```python
from build123d import *

# Parameters (mm, degrees)
SKETCH1_W           = 97.3
SKETCH1_H           = 47
BOSS_EXTRUDE1_DEPTH = 1.6
SKETCH2_W           = 12.310757006
SKETCH2_H           = 2.521357674
SKETCH2_W_2         = 11.997879532
BOSS_EXTRUDE2_DEPTH = 20
SKETCH3_R           = 1.016
SKETCH3_R_2         = 1.316
CUT_EXTRUDE3_DEPTH  = 2.6


with BuildPart() as part:
    # Sketch1 → Boss-Extrude1 (new body)
    with BuildSketch(Plane(origin=(0, 0, 0), x_dir=(1, 0, 0), z_dir=(0, 1, 0))):
        with Locations((48.65, -23.5)):
            Rectangle(SKETCH1_W, SKETCH1_H)
    extrude(amount=BOSS_EXTRUDE1_DEPTH)

    # Sketch2 → Boss-Extrude2 (add)
    with BuildSketch(Plane(origin=(0, 1.6, 0), x_dir=(1, 0, 0), z_dir=(0, 1, 0))):
        with Locations((17.456098962, -45.739321163)):
            Rectangle(SKETCH2_W, SKETCH2_H)
        with Locations((66.019073535, -45.739321163)):
            Rectangle(SKETCH2_W_2, SKETCH2_H)
    extrude(amount=BOSS_EXTRUDE2_DEPTH)

    # Sketch3 → Cut-Extrude3 (cut, through all)
    with BuildSketch(Plane(origin=(0, 1.6, 0), x_dir=(1, 0, 0), z_dir=(0, 1, 0))):
        with Locations((3.16, -3.81)):
            Circle(SKETCH3_R)
        with Locations((93.617, -3.81)):
            Circle(SKETCH3_R)
        with Locations((93.744, -43.916)):
            Circle(SKETCH3_R_2)
        with Locations((3.16, -43.916)):
            Circle(SKETCH3_R)
    extrude(amount=-CUT_EXTRUDE3_DEPTH, mode=Mode.SUBTRACT)


solid = part.part
```
Check sheet for the modelled part. Datum: model origin and axes. Units: mm. A direction names the side the tool comes from. Round coordinates to 2 decimals unless told otherwise and drop trailing zeros. Loops run counter-clockwise (first coordinate to the right, second up) from the corner with the lowest first, then second, coordinate; pieces in that order, holes last. Notation, with made-up numbers: M 23.5,37 L 42.5,37 A8 ccw 42.5,46 Z; hole C -19.75,59 d1. An arc over 180 degrees is marked long. Answer as a JSON object with one key per item and string values.
1. Access from +Z, -Z, +X, -X, +Y, -Y to the whole of each face (thin tool, end or side, straight path). Record for faces 4 (the flat face through (11.301, 11, 46)), 5 (the flat face through (17, 11, 44.479)), 6 (the flat face through (72.018, 11, 46)).
Reply:
{"face 4": "+Z, -Z, -X, +Y", "face 5": "-Z, +X, -X, +Y", "face 6": "+Z, -Z, +X, +Y"}
2. Scan lines: line 1 (Z direction, x = 3.16, y = 1.2); line 2 (X direction, y = 0.65, z = 3.81); line 3 (Y direction, x = 21.5, z = 9.5). Record each from-to range of solid material in increasing order.
Reply:
{"line 1": "z = 0 to 2.79, 4.83 to 42.9, 44.93 to 47", "line 2": "x = 0 to 2.14, 4.18 to 92.6, 94.63 to 97.3", "line 3": "y = 0 to 1.6"}
3. Gauge pin test, flat ends, axial feed: P1, Ø1.3, axis at y = 16, z = 45.5, coming from the -X side; P2, Ø5, axis at x = 28.5, z = 30.5, coming from the +Y side; P3, Ø10, axis at y = 14.5, z = 40, coming from the +X side. Record the tip position at first contact, or that the pin passes through.
Reply:
{"P1": "stops at x = 11.3", "P2": "stops at y = 1.6", "P3": "stops at x = 72.02"}
4. Section check C-C (z = 3.81). Record the boundary of the cut face in (x, y).
Reply:
{"outline": "M 0,0 L 2.14,0 L 2.14,1.6 L 0,1.6 Z; M 4.18,0 L 92.6,0 L 92.6,1.6 L 4.18,1.6 Z; M 94.63,0 L 97.3,0 L 97.3,1.6 L 94.63,1.6 Z"}
5. Section check D-D (x = 35.5). Record the boundary of the cut face in (y, z), plus the area to 3 significant figures.
Reply:
{"outline": "M 0,0 L 1.6,0 L 1.6,47 L 0,47 Z", "area": "75.2 mm²"}
6. Mould release check, pull along Z, two halves, no side actions. Record for faces 1 (the flat face through (48, 1.6, 23)), 2 (the flat face through (41, 1, 47)), 3 (the cylindrical face through (92.81, 0.81, 4.43)): pulls with the +Z half, pulls with the -Z half, needs draft (parallel to the pull), parting line crosses it, or undercut.
Reply:
{"face 1": "needs draft", "face 2": "pulls with the +Z half", "face 3": "undercut"}
7. Section check B-B (y = 20). Record the boundary of the cut face in (x, z), plus the area to 3 significant figures.
Reply:
{"outline": "M 11.3,44.48 L 23.61,44.48 L 23.61,47 L 11.3,47 Z; M 60.02,44.48 L 72.02,44.48 L 72.02,47 L 60.02,47 Z", "area": "61.3 mm²"}
8. Section check A-A (x = 3.16). Record the boundary of the cut face in (y, z).
Reply:
{"outline": "M 0,0 L 1.6,0 L 1.6,2.79 L 0,2.79 Z; M 0,4.83 L 1.6,4.83 L 1.6,42.9 L 0,42.9 Z; M 0,44.93 L 1.6,44.93 L 1.6,47 L 0,47 Z"}
